```python
from build123d import *

# Parameters (mm, degrees)
F0_W     = 44
F0_H     = 69
F1_DEPTH = 350
F2_W     = 25
F2_H     = 50
F3_DEPTH = 44.001
F4_W     = 10
F4_H     = 350
F5_DEPTH = 100


with BuildPart() as f1:
    # F0 (on Top) → F1 (new body)
    with BuildSketch(Plane.XY):
        Rectangle(F0_W, F0_H)
    extrude(amount=F1_DEPTH)

    # F2 (on face) → F3 (cut, through all)
    with BuildSketch(Plane.YZ.offset(22)):
        Polygon((-10.5, 85), (34.5, 85), (34.5, 175), (34.5, 265), (-10.5, 265), (-10.5, 175), align=None)
        with Locations((22, 25)):
            Rectangle(F2_W, F2_H)
        with Locations((22, 325)):
            Rectangle(F2_W, F2_H)
    extrude(amount=-F3_DEPTH, mode=Mode.SUBTRACT)

    # F4 (on face) → F5 (cut)
    with BuildSketch(Plane.YZ.offset(22)):
        with Locations((-29.5, 175)):
            Rectangle(F4_W, F4_H)
    extrude(amount=-F5_DEPTH, mode=Mode.SUBTRACT)


solid = f1.part
```
Can you work these out from the model? Positions are in its coordinate system, mm. A direction names the side the tool comes from. Coordinates: 2 decimals unless noted, no trailing zeros. Loops run counter-clockwise (first coordinate to the right, second up) from the corner with the lowest first, then second, coordinate; pieces in that order, holes last.
1) For pin 1 (5 mm diameter, centred on x = 8, z = 94.5, fed in from +Y); pin 2 (12.5 mm diameter, centred on x = -4, y = 17, fed in from +Z); pin 3 (13 mm diameter, centred on x = -8.5, y = 17.5, fed in from -Z), each with a flat end and sliding along its axis, tell me the tip position at first contact or that it passes through.
2) Which directions (+Z, -Z, +X, -X, +Y, -Y) give clear straight access to the entire face, cutting with the end or side of a thin tool? Please do faces 5 (the flat face through (0, 22, 300)), 6 (the flat face through (0, 9.5, 25)), 7 (the flat face through (0, 12, 265)), 8 (the flat face through (-22, -15, 173)).
3) Imagine slicing it at C-C on y = 24.5. List the corners of the cut face in (x, z) for me.
4) I need wall thicknesses on probe 1 along Z at (x, y) = (-4, -8.5); probe 2 along Z at (x, y) = (-19, 24.5); probe 3 along Y at (x, z) = (4.5, 156). Which ranges of each line are inside material? Lowest first, please.
5) Imagine slicing it at D-D on z = 156. List the corners of the cut face in (x, y) for me.
6) Imagine slicing it at A-A on y = -2. List the corners of the cut face in (x, z) for me.
7) Thinking about a two-plate mould opening in Z: for faces 1 (the flat face through (0, -10.5, 176)), 2 (the flat face through (0, -7, 350)), 3 (the flat face through (0, 34.5, 67)), 4 (the flat face through (0, 12, 85)), which applies, pulls with the +Z half, pulls with the -Z half, needs draft (parallel to the pull), parting line crosses it, or undercut?
8) Imagine slicing it at B-B on x = 17. List the corners of the cut face in (y, z) for me.
Completed:
1. pin 1: stops at y = -10.5
1. pin 2: stops at z = 300
1. pin 3: stops at z = 50
2. face 5: +Z, +X, -X, +Y
2. face 6: -Z, +X, -X, +Y
2. face 7: +X, -X, +Y
2. face 8: +Z, -Z, -X, +Y, -Y
3. outline: (-22, 50) - (22, 50) - (22, 85) - (-22, 85) - close; (-22, 265) - (22, 265) - (22, 300) - (-22, 300) - close
4. probe 1: z = 0 to 85, 265 to 350
4. probe 2: z = 50 to 85, 265 to 300
4. probe 3: y = -24.5 to -10.5
5. outline: (-22, -24.5) - (22, -24.5) - (22, -10.5) - (-22, -10.5) - close
6. outline: (-22, 0) - (22, 0) - (22, 85) - (-22, 85) - close; (-22, 265) - (22, 265) - (22, 350) - (-22, 350) - close
7. face 1: undercut
7. face 2: pulls with the +Z half
7. face 3: needs draft
7. face 4: undercut
8. outline: (-24.5, 0) - (9.5, 0) - (9.5, 50) - (34.5, 50) - (34.5, 85) - (-10.5, 85) - (-10.5, 265) - (34.5, 265) - (34.5, 300) - (9.5, 300) - (9.5, 350) - (-24.5, 350) - close
